Design review of the part built by this model. Coordinates are the model's own, in mm. A direction names the side the tool comes from. Round coordinates to 2 decimals unless told otherwise and drop trailing zeros. Order: outer loops, then holes, each group sorted by start corner. A loop starts at its lowest first (then second) coordinate and runs counter-clockwise, first axis right, second up. Notation, with made-up numbers: (37, 71.5) - (83, 71.5) arc R25 cw to (83, 87.5) - close; hole circle Ø5 at (72, 64). An arc over 180 degrees is marked (long way). Use CSV: the item, a comma, the result in double quotes.
from build123d import *

# Parameters (mm, degrees)
SALIENTE_EXTRUIR1_START = -7
CROQUIS1_R              = 6
SALIENTE_EXTRUIR1_DEPTH = 4
CROQUIS2_R              = 6
SALIENTE_EXTRUIR2_DEPTH = 3
CROQUIS3_R              = 9
SALIENTE_EXTRUIR3_DEPTH = 3
CROQUIS4_R              = 1.6
CORTAR_EXTRUIR1_DEPTH   = 11.5
CROQUIS5_R              = 3
CORTAR_EXTRUIR2_DEPTH   = 3
REDONDEO1_R             = 2


with BuildPart() as part:
    # Croquis1 → Saliente-Extruir1 (new body)
    with BuildSketch(Plane(origin=(0, 0, 34.55), x_dir=(-1, 0, 0), z_dir=(0, 0, -1)).offset(SALIENTE_EXTRUIR1_START)):
        with Locations((13.509321031, -3.657231325)):
            Circle(CROQUIS1_R)
        Polygon((9.359321031, -1.261227707), (9.359321031, -6.053234942), (13.509321031, -8.449238559), (17.659321031, -6.053234942), (17.659321031, -1.261227707), (13.509321031, 1.13477591), align=None, mode=Mode.SUBTRACT)
    extrude(amount=SALIENTE_EXTRUIR1_DEPTH)

    # Croquis2 → Saliente-Extruir2 (add)
    with BuildSketch(Plane(origin=(0, 0, 37.55), x_dir=(-1, 0, 0), z_dir=(0, 0, -1))):
        with Locations((13.509321031, -3.657231325)):
            Circle(CROQUIS2_R)
    extrude(amount=SALIENTE_EXTRUIR2_DEPTH)

    # Croquis3 → Saliente-Extruir3 (add)
    with BuildSketch(Plane(origin=(0, 0, 34.55), x_dir=(-1, 0, 0), z_dir=(0, 0, -1))):
        with Locations((13.509321031, -3.657231325)):
            Circle(CROQUIS3_R)
    extrude(amount=SALIENTE_EXTRUIR3_DEPTH)

    # Croquis4 → Cortar-Extruir1 (cut)
    with BuildSketch(Plane(origin=(0, 0, 31.55), x_dir=(-1, 0, 0), z_dir=(0, 0, -1))):
        with Locations((13.509321031, -3.657231325)):
            Circle(CROQUIS4_R)
    extrude(amount=-CORTAR_EXTRUIR1_DEPTH, mode=Mode.SUBTRACT)

    # Croquis5 → Cortar-Extruir2 (cut)
    with BuildSketch(Plane(origin=(0, 0, 31.55), x_dir=(-1, 0, 0), z_dir=(0, 0, -1))):
        with Locations((13.509321031, -3.657231325)):
            Circle(CROQUIS5_R)
    extrude(amount=-CORTAR_EXTRUIR2_DEPTH, mode=Mode.SUBTRACT)

    # Redondeo1
    redondeo1_edges = [part.edges().sort_by_distance(p)[0] for p in [
        (-4.509321031, -3.657231325, 31.55),
    ]]
    fillet(redondeo1_edges, radius=REDONDEO1_R)


solid = part.part
1) We need section A-A (z = 39.25). Give the boundary of the cut face in (x, y), then the cut area to 3 significant figures.
Data:
outline,"circle Ø12 at (-13.51, -3.66); hole (-17.66, -6.05) - (-13.51, -8.45) - (-9.36, -6.05) - (-9.36, -1.26) - (-13.51, 1.13) - (-17.66, -1.26) - close"
area,"53.4 mm2"
2) The part is to be moulded in two halves that separate along Y. For faces 4 (the face through (-15, -10, 34.55)), 5 (the face through (-22.094, -0.954, 34.057)), 6 (the face through (-11.46, -0.05, 39.58)), say which applies: +Y half, -Y half, draft (parallel to the pull), parting line (faces both ways), or undercut.
Data:
face 4,"draft"
face 5,"parting line"
face 6,"undercut"
3) To check wall thickness, follow L1, parallel to X at y = -2.75, z = 33.5; L2, parallel to Z at x = -9, y = 1.5; L3, parallel to Z at x = -14.25, y = -7. State the ranges of each line that lie inside material, in increasing order. Write a range as from..to.
Data:
L1,"x = -22.46..-16.37, -10.65..-4.56"
L2,"z = 31.55..34.55"
L3,"z = 31.55..37.55"
4) We need section B-B (z = 32.5). Give the boundary of the cut face in (x, y), then the cut area to 3 significant figures.
Data:
outline,"circle Ø17.4 at (-13.51, -3.66); hole circle Ø6 at (-13.51, -3.66)"
area,"210 mm2"
5) For faces 1 (the face through (-15, -5, 34.55)), 2 (the face through (-7.515, -3.393, 38.099)), 3 (the face through (-14.37, -2.31, 36.03)), list the 3-axis set-ups (+Z, -Z, +X, -X, +Y, -Y) from which the entire face can be reached by the end or side of a thin tool; tool diameter is ignored.
Data:
face 1,"-Z"
face 2,"+Z"
face 3,"+Z, -Z"
6) Insertion check: pin 1 Ø4.5 at (y, z) = (-2.5, 39.5) entering from -X; pin 2 Ø3.5 at (x, y) = (-13.51, -3.66) entering from +Z; pin 3 Ø1.5 at (x, z) = (-18.5, 38) entering from -Y; pin 4 Ø1.9 at (x, y) = (-13.51, -3.66) entering from +Z. Each pin has a flat end and moves straight along its axis. Give the tip position at first contact, or say it passes through.
Data:
pin 1,"stops at x = -19.51"
pin 2,"stops at z = 37.55"
pin 3,"stops at y = -7.9"
pin 4,"passes through"
7) We need section C-C (z = 36.75). Give the boundary of the cut face in (x, y).
Data:
outline,"circle Ø12 at (-13.51, -3.66); hole circle Ø3.2 at (-13.51, -3.66)"
